from build123d import *

# Parameters (mm, degrees)
F0_R      = 20
F1_DEPTH  = 10
F3_DEPTH  = 25
F4_DEPTH  = 25
F6_DEPTH  = 25
F7_W      = 35.777088
F7_H      = 2
F8_DEPTH  = 8
F9_W      = 2
F9_H      = 17.974984
F10_DEPTH = 2
F11_R     = 4
F12_DEPTH = 2
F13_R     = 1
F14_DEPTH = 25


with BuildPart() as f1:
    # F0 (on Top) → F1 (new body)
    with BuildSketch(Plane.XY):
        Circle(F0_R)
    extrude(amount=F1_DEPTH)

    # F2 (on face) → F3 (cut)
    with BuildSketch(Plane.XY.offset(10)):
        with BuildLine():
            Line((-20, 0), (0, 0))
            Line((0, 0), (20, 0))
            ThreePointArc((20, 0), (0, 20), (-20, 0))
        make_face()
    extrude(amount=-F3_DEPTH, mode=Mode.SUBTRACT)

    # F2 (on face) → F4 (cut)
    with BuildSketch(Plane.XY.offset(10)):
        with BuildLine():
            Line((-20, 0), (0, 0))
            Line((0, 0), (20, 0))
            ThreePointArc((20, 0), (0, 20), (-20, 0))
        make_face()
    extrude(amount=-F4_DEPTH, mode=Mode.SUBTRACT)

    # F5 (on face) → F6 (cut)
    with BuildSketch(Plane.XY.offset(10)):
        with BuildLine():
            ThreePointArc((-17.888544, -2), (0, -18), (17.888544, -2))
            Line((17.888544, -2), (-17.888544, -2))
        make_face()
    extrude(amount=-F6_DEPTH, mode=Mode.SUBTRACT)

    # F7 (on face) → F8 (cut)
    with BuildSketch(Plane(origin=(0, 0, 0), x_dir=(1, 0, 0), z_dir=(0, 0, -1))):
        with Locations((0, 1)):
            Rectangle(F7_W, F7_H)
    extrude(amount=-F8_DEPTH, mode=Mode.SUBTRACT)

    # F9 (on face) → F10 (join)
    with BuildSketch(Plane.XY.offset(10)):
        with Locations((0, -10.987492)):
            Rectangle(F9_W, F9_H)
    extrude(amount=-F10_DEPTH)

    # F11 (on face) → F12 (join)
    with BuildSketch(Plane.XY.offset(10)):
        Circle(F11_R)
    extrude(amount=-F12_DEPTH)

    # F13 (on face) → F14 (cut)
    with BuildSketch(Plane.XY.offset(10)):
        Circle(F13_R)
    extrude(amount=-F14_DEPTH, mode=Mode.SUBTRACT)


solid = f1.part
Work out the finished part from the listing and answer in its coordinate system (mm). A direction names the side the tool comes from. Give positions to 0.01 mm unless a question says otherwise; leave off trailing zeros. Write each loop counter-clockwise with the first axis right and the second up, starting at its lowest first coordinate (ties: lowest second). Pieces come first, ordered by that corner, then holes.
Q1. A tool of negligible diameter and unlimited length cuts with its end or side. For faces 1 (the face through (-15, 0, 9)), 2 (the face through (14, 0, 9)), 3 (the face through (17.889, -1, 4)), 4 (the face through (2.4, -3.2, 9)), from which of +Z, -Z, +X, -X, +Y, -Y can it reach the whole face along a straight path? Write none if from no direction.
Answer:
face 1: +Z, -Z, -X, +Y
face 2: +Z, -Z, +X, +Y
face 3: -Z, +Y
face 4: +Z, -Z
Q2. Given pin 1 (6 mm diameter, centred on x = 8, z = 2.5, fed in from +Y); pin 2 (2 mm diameter, centred on x = -13, z = 1.5, fed in from +Y); pin 3 (2 mm diameter, centred on x = 8.5, z = 9.5, fed in from -Y), each flat-ended and moving along its own axis, determine where each tip first touches the part or whether it passes through.
Answer:
pin 1: stops at y = -14.25
pin 2: stops at y = -11.31
pin 3: stops at y = -18.54
Q3. The part is cut by section A-A on x = 0. Give the vertices of the cut face in (y, z), and give its area (3 significant figures).
Answer:
outline: (-20, 0) - (-18, 0) - (-18, 8) - (-1, 8) - (-1, 10) - (-20, 10) - close; (1, 8) - (4, 8) - (4, 10) - (1, 10) - close
area: 60.0 mm2
Q4. The part is cut by section D-D on x = -11. Give the vertices of the cut face in (y, z).
Answer:
outline: (-16.7, 0) - (-14.25, 0) - (-14.25, 10) - (-16.7, 10) - close; (-2, 8) - (0, 8) - (0, 10) - (-2, 10) - close
Q5. The part is cut by section C-C on z = 1.75. Give the vertices of the cut face in (x, y).
Answer:
outline: (-20, 0) arc R20 ccw to (20, 0) - (17.89, 0) - (17.89, -2) arc R18 cw to (-17.89, -2) - (-17.89, 0) - close
Q6. Straight lines are drawn through the part: L1, parallel to Y at x = 0, z = 9.1; L2, parallel to X at y = -9.75, z = 8.5; L3, parallel to X at y = -5, z = 9.75. For each, find the intervals that lie inside material, in ascending order.
Answer:
L1: y = -20 to -1, 1 to 4
L2: x = -17.46 to -15.13, -1 to 1, 15.13 to 17.46
L3: x = -19.36 to -17.29, -1 to 1, 17.29 to 19.36
Q7. The part is cut by section B-B on y = -15.5. Give the vertices of the cut face in (x, z).
Answer:
outline: (-12.64, 0) - (-9.15, 0) - (-9.15, 10) - (-12.64, 10) - close; (-1, 8) - (1, 8) - (1, 10) - (-1, 10) - close; (9.15, 0) - (12.64, 0) - (12.64, 10) - (9.15, 10) - close
Q8. For a pull along X with two mould halves and no side action, classify faces 5 (the face through (0, -6, 10)), 6 (the face through (-17.889, -1, 4)), 7 (the face through (0, -3, 8)), 8 (the face through (0, -20, 5)) as released by +X, released by -X, zero draft, split by the parting line, or undercut.
Answer:
face 5: zero draft
face 6: undercut
face 7: undercut
face 8: split by the parting line
